Could you check a few things on this model? Use its own coordinates, in mm. Round coordinates to 2 decimals unless told otherwise and drop trailing zeros. Loops run counter-clockwise (first coordinate to the right, second up) from the corner with the lowest first, then second, coordinate; pieces in that order, holes last.
Autodesk Fusion 360 part; units mm, degrees
sketch "Sketch1" plane through (0, 0, 0) normal (0, 0, 1) x (1, 0, 0)
  circle A0 centre (0, 0) radius 5
  circle A1 centre (0, 0) radius 3.95
  dimension "d1" = 10
  dimension "d2" = 7.9
extrude "Extrude1" add sketch "Sketch1" along normal blind 2 contours A0 | A1
extrude "Extrude2" add sketch "Sketch1" along normal blind 21
fillet "Fillet1" radius 2 1 edges at (-4.6616, -1.8081, 0)
Item 1: If we section it at A-A, the plane y = 0: Please give me the cut outline in (x, z), then the cut area to 3 significant figures.
Results list:
outline: (-5, 2) arc R2 ccw to (-3, 0) - (3, 0) arc R2 ccw to (5, 2) - (5, 21) - (3.95, 21) - (3.95, 2) - (-3.95, 2) - (-3.95, 21) - (-5, 21) - close
area: 58.2 mm2
Item 2: Will these pins go through, and if not, where does the flat tip stop? pin 1 (1.5 mm diameter, centred on y = 3, z = 15, fed in from -X); pin 2 (1 mm diameter, centred on x = 2, y = 4, fed in from -Z); pin 3 (2.5 mm diameter, centred on x = -1.5, y = 2, fed in from +Z).
Results list:
pin 1: stops at x = -4.47
pin 2: stops at z = 0.25
pin 3: stops at z = 2
Item 3: If we section it at B-B, the plane z = 13: Please give me the cut outline in (x, y).
Results list:
outline: circle Ø10 at (0, 0); hole circle Ø7.9 at (0, 0)
Item 4: If I drill on line 1 along Y through (x, z) = (0, 14.25); line 2 along Z through (x, y) = (0, 1.5); line 3 along X through (y, z) = (2.25, 6.5), over which ranges is the centre line in solid material (lowest first)?
Results list:
line 1: y = -5 to -3.95, 3.95 to 5
line 2: z = 0 to 2
line 3: x = -4.47 to -3.25, 3.25 to 4.47
Item 5: We'd pull the mould along Y, two halves only. Please class faces 1 (the cylindrical face through (-3.135, 2.404, 11.367)), 2 (the flat face through (0, 0, 2)), 3 (the cylindrical face through (-1.08, 4.88, 11.37)), 4 (the flat face through (0, 0, 0)): released by +Y, released by -Y, zero draft, split by the parting line, or undercut.
Results list:
face 1: undercut
face 2: undercut
face 3: split by the parting line
face 4: zero draft
